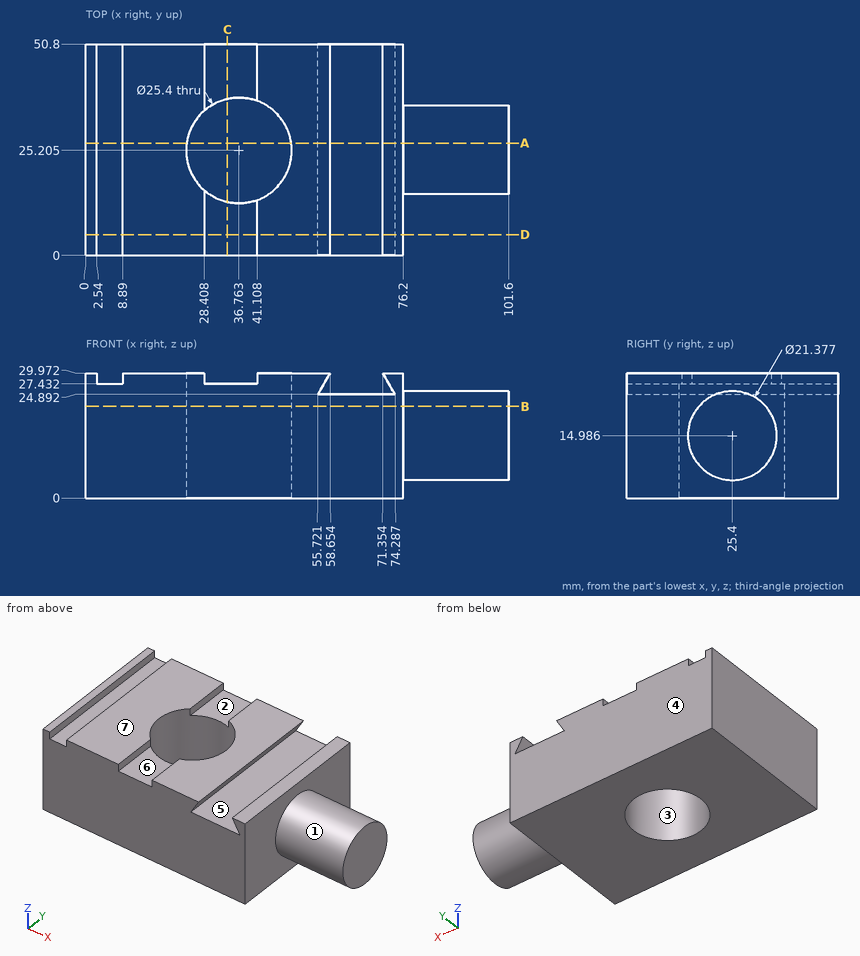
The drawing under review shows one solid part. Ordinate dimensions are in mm from its lowest x, y, z. A direction names the side the tool comes from. Give positions to 0.01 mm unless a question says otherwise; leave off trailing zeros. Write each loop counter-clockwise with the first axis right and the second up, starting at its lowest first coordinate (ties: lowest second). Pieces come first, ordered by that corner, then holes. Notation, with made-up numbers: (79, 86.5) - (109, 86.5) arc R21 ccw to (109, 95.5) - close; hole circle Ø9 at (48, 57.5). An arc over 180 degrees is marked (long way). Answer in a Markdown table with one row per item. Add a question column.
1. We need section D-D on y = 5. Write out the cut boundary in (x, z), then the cut area to 3 significant figures.
2. Tool access review of the marked faces 5, 6 and 7: name each direction out of +Z, -Z, +X, -X, +Y, -Y from which nothing blocks a thin tool from reaching the whole face with its end or side.
3. We need section A-A on y = 27. Write out the cut boundary in (x, z) (1 decimal).
4. Insertion check: P1, Ø10, axis at y = 9.5, z = 25.5, coming from the -X side; P2, Ø15, axis at x = 36.76, y = 25.21, coming from the -Z side; P3, Ø8, axis at y = 12.5, z = 26.5, coming from the +X side; P4, Ø3, axis at x = 31.5, y = 9, coming from the +Z side. Each pin has a flat end and moves straight along its axis. Give the tip position at first contact, or say it passes through.
5. Wall thickness on line 1 along X through (y, z) = (14, 25) (1 decimal); line 2 along X through (y, z) = (25, 12) (1 decimal); line 3 along Z through (x, y) = (64, 45): over which ranges is each line inside the solid? List them lowest first. Write a range as [from, to].
6. Draft analysis for pull direction Y (two halves, no side actions). For the marked faces 1, 2, 3 and 4, state which applies: +Y half, -Y half, draft (parallel to the pull), parting line (faces both ways), or undercut.
7. We need section C-C on x = 34. Write out the cut boundary in (y, z).
8. We need section B-B on z = 22. Write out the cut boundary in (x, y) (1 decimal).
Ans:
| question | item | result |
|---|---|---|
| 1 | outline | (0, 0) - (76.2, 0) - (76.2, 29.97) - (71.35, 29.97) - (74.29, 24.89) - (55.72, 24.89) - (58.65, 29.97) - (41.11, 29.97) - (41.11, 27.43) - (28.41, 27.43) - (28.41, 29.97) - (8.89, 29.97) - (8.89, 27.43) - (2.54, 27.43) - (2.54, 29.97) - (0, 29.97) - close |
| 1 | area | 2,160 mm^2 |
| 2 | face 5 | +Y, -Y |
| 2 | face 6 | +Z, +Y, -Y |
| 2 | face 7 | +Z, +X, -X, +Y, -Y |
| 3 | outline | (0, 0) - (24.2, 0) - (24.2, 30) - (8.9, 30) - (8.9, 27.4) - (2.5, 27.4) - (2.5, 30) - (0, 30) - close; (49.3, 0) - (76.2, 0) - (76.2, 4.4) - (101.6, 4.4) - (101.6, 25.6) - (76.2, 25.6) - (76.2, 30) - (71.4, 30) - (74.3, 24.9) - (55.7, 24.9) - (58.7, 30) - (49.3, 30) - close |
| 4 | P1 | stops at x = 0 |
| 4 | P2 | passes through |
| 4 | P3 | stops at x = 76.2 |
| 4 | P4 | stops at z = 27.43 |
| 5 | line 1 | x = [0, 30.8], [42.7, 55.8], [74.2, 76.2] |
| 5 | line 2 | x = [0, 24.1], [49.5, 101.6] |
| 5 | line 3 | z = [0, 24.89] |
| 6 | face 1 | parting line |
| 6 | face 2 | draft |
| 6 | face 3 | undercut |
| 6 | face 4 | +Y half |
| 7 | outline | (0, 0) - (12.81, 0) - (12.81, 27.43) - (0, 27.43) - close; (37.6, 0) - (50.8, 0) - (50.8, 27.43) - (37.6, 27.43) - close |
| 8 | outline | (0, 0) - (76.2, 0) - (76.2, 17.3) - (101.6, 17.3) - (101.6, 33.5) - (76.2, 33.5) - (76.2, 50.8) - (0, 50.8) - close; hole circle Ø25.4 at (36.8, 25.2) |
